Geometry: final body of the model. Coordinates: model frame, mm. A direction names the side the tool comes from. Give positions to 0.01 mm unless a question says otherwise; leave off trailing zeros. Order: outer loops, then holes, each group sorted by start corner. A loop starts at its lowest first (then second) coordinate and runs counter-clockwise, first axis right, second up. Notation, with made-up numbers: (12, 40) -> (65, 40) arc R22 ccw to (65, 61) -> close; hole circle Ø7 at (82, 40.5). An arc over 180 degrees is marked (long way). Answer in a Markdown table with one row per item. Add a question column.
Q1. Cut plane B-B on x = 3. Return the cut outline in (y, z), and give its area (3 significant figures).
Q2. Set-up query: faces 1 (the face through (25, 26, -22)), 2 (the face through (15, -9, -10)), 3 (the face through (0, 30, 22)). Return all of +Z, -Z, +X, -X, +Y, -Y with unobstructed straight access to the full face (end or side cutting, diameter ignored); none if empty.
Q3. Cut plane C-C on y = 25. Return the cut outline in (x, z).
Q4. Pull-direction query (Y, two-part tool) for faces 4 (the face through (10, 53, -21)), 5 (the face through (0, 25, 24.365)), 6 (the face through (-15, 59, -10)); classes: +Y half, -Y half, draft (parallel to the pull), parting line (faces both ways), or undercut.
Q5. Line query: line 1 along X through (y, z) = (25.5, -45); line 2 along Z through (x, y) = (9, 25); line 3 along Z through (x, y) = (0.5, 25). Output: solid intervals per line, ascending. Write a range as from..to.
Q6. Cut plane D-D on z = 38. Return the cut outline in (x, y), and give its area (3 significant figures).
Q7. Cut plane A-A on z = 0. Return the cut outline in (x, y), and give its area (3 significant figures).
Q8. Contact query for flat-ended pins moving along their axis: P1, Ø5, axis at x = -19, z = 7, coming from the +Y side; P2, Ø4, axis at x = -8.5, z = 22, coming from the +Y side; P3, Ø5.5, axis at x = 11.5, z = 22, coming from the -Y side. Output: stop coordinate, or through.
from build123d import *

# Parameters (mm, degrees)
F3_DEPTH = 50


with BuildPart() as f1:
    # F0 (on Top) → F1 (revolve)
    with BuildSketch(Plane.XY):
        Polygon((15, -25), (25, -25), (25, 25), (-25, 25), (-25, -25), (-15, -25), (-15, -10), (-5, -10), (-5, -25), (5, -25), (5, -10), (15, -10), align=None)
    revolve(axis=Axis((0, 25, 0), (-1, 0, 0)))

    # F2 (on face) → F3 (cut)
    with BuildSketch(Plane.YZ.offset(25)):
        with BuildLine():
            Line((20, 24.364917), (20, 19.364917))
            ThreePointArc((20, 19.364917), (25, -20), (30, 19.364917))
            Line((30, 19.364917), (30, 24.364917))
            Line((30, 24.364917), (25, 24.364917))
            Line((25, 24.364917), (20, 24.364917))
        make_face()
    extrude(amount=-F3_DEPTH, mode=Mode.SUBTRACT)


solid = f1.part
Completed:
| question | item | result |
|---|---|---|
| 1 | outline | circle Ø100 at (25, 0); hole (20, 19.36) arc R20 ccw (long way) to (30, 19.36) -> (30, 24.36) -> (20, 24.36) -> close |
| 1 | area | 6,550 mm² |
| 2 | face 1 | +Z, -Z, +X, +Y, -Y |
| 2 | face 2 | none |
| 2 | face 3 | +X, -X |
| 3 | outline | (-25, -50) -> (-15, -50) -> (-15, -35) -> (-5, -35) -> (-5, -50) -> (5, -50) -> (5, -35) -> (15, -35) -> (15, -50) -> (25, -50) -> (25, -20) -> (-25, -20) -> close; (-25, 24.36) -> (25, 24.36) -> (25, 50) -> (15, 50) -> (15, 35) -> (5, 35) -> (5, 50) -> (-5, 50) -> (-5, 35) -> (-15, 35) -> (-15, 50) -> (-25, 50) -> close |
| 4 | face 4 | parting line |
| 4 | face 5 | undercut |
| 4 | face 6 | draft |
| 5 | line 1 | x = -25..-15, -5..5, 15..25 |
| 5 | line 2 | z = -35..-20, 24.36..35 |
| 5 | line 3 | z = -50..-20, 24.36..50 |
| 6 | outline | (-25, -7.5) -> (-15, -7.5) -> (-15, 57.5) -> (-25, 57.5) -> close; (-5, -7.5) -> (5, -7.5) -> (5, 57.5) -> (-5, 57.5) -> close; (15, -7.5) -> (25, -7.5) -> (25, 57.5) -> (15, 57.5) -> close |
| 6 | area | 1,950 mm² |
| 7 | outline | (-25, -25) -> (-15, -25) -> (-15, -10) -> (-5, -10) -> (-5, -25) -> (5, -25) -> (5, -10) -> (15, -10) -> (15, -25) -> (25, -25) -> (25, 5) -> (-25, 5) -> close; (-25, 45) -> (25, 45) -> (25, 75) -> (15, 75) -> (15, 60) -> (5, 60) -> (5, 75) -> (-5, 75) -> (-5, 60) -> (-15, 60) -> (-15, 75) -> (-25, 75) -> close |
| 7 | area | 2,400 mm² |
| 8 | P1 | stops at y = 74.8 |
| 8 | P2 | stops at y = 53.72 |
| 8 | P3 | stops at y = -4.23 |
